Here's how the part is built. I have some questions about the finished solid (model axes, mm). Face numbers are marked on the shaded views. A direction names the side the tool comes from. Coordinates: 2 decimals unless noted, no trailing zeros. Write each loop counter-clockwise with the first axis right and the second up, starting at its lowest first coordinate (ties: lowest second). Pieces come first, ordered by that corner, then holes. Notation, with made-up numbers: (55.5, -36.5) -> (65.5, -36.5) arc R29 ccw to (65.5, 2.5) -> close; hole circle Ø6 at (30.5, 62.25). An arc over 180 degrees is marked (long way). Put each result on its own line as item: value. Start each with the question number.
Item 1: I want a section at C-C, the plane y = 33. List the corners of the cut face in (x, z) for me, then the cut area to 3 significant figures.
Item 2: If we mould it in two halves opening along X, with no side actions, what happens to the marked faces 1, 2 and 3? For each: released by +X, released by -X, zero draft, split by the parting line, or undercut.
Item 3: I want a section at D-D, the plane y = 109.5. State how many separate pieces and enclosed holes the cut face has, then the cut area to 3 significant figures.
Item 4: On a 3-axis mill with a long thin cutter (end or side, diameter ignored), from which of +Z, -Z, +X, -X, +Y, -Y can I reach the whole of each face in a straight line? I mean the marked faces 4, 5, 6, 7 and 8. Say none if no direction works.
Item 5: I want a section at B-B, the plane x = 0. List the corners of the cut face in (y, z) for me.
Item 6: I want a section at A-A, the plane z = 0. List the corners of the cut face in (x, y) for me.
Item 7: I need wall thicknesses on line 1 (Z direction, x = -29, y = 67.5); line 2 (X direction, y = 96, z = 9); line 3 (Y direction, x = 53.6, z = 0). Which ranges of each line are inside material? Lowest first, please. Write a range as [from, to].
Item 8: For pin 1 (21 mm diameter, centred on x = -39, z = 29.5, fed in from -Y); pin 2 (5 mm diameter, centred on x = 9, z = -22, fed in from -Y); pin 3 (4 mm diameter, centred on x = -42.5, z = -30.5, fed in from +Y); pin 4 (21.5 mm diameter, centred on y = 103.98, z = 0, fed in from +X), each with a flat end and sliding along its axis, tell me the tip position at first contact or that it passes through.
from build123d import *

# Parameters (mm, degrees)
SKETCH1_W           = 110
SKETCH1_H           = 90
SKETCH1_W_2         = 106
SKETCH1_H_2         = 86
BOSS_EXTRUDE1_DEPTH = 80
SKETCH2_W           = 110
SKETCH2_H           = 90
BOSS_EXTRUDE2_DEPTH = 2
BOSS_EXTRUDE3_DEPTH = 40
CUT_EXTRUDE1_DEPTH  = 40
BOSS_EXTRUDE4_DEPTH = 2
SKETCH11_W          = 23
SKETCH11_H          = 13
CUT_EXTRUDE2_DEPTH  = 13
REVOLVE_THIN3_ANGLE = 180
SKETCH13_R          = 12
CUT_EXTRUDE3_DEPTH  = 97
SKETCH14_R          = 12
CUT_EXTRUDE4_DEPTH  = 112


with BuildPart() as part:
    # Sketch1 → Boss-Extrude1 (new body)
    with BuildSketch(Plane(origin=(0, 0, 0), x_dir=(1, 0, 0), z_dir=(0, 1, 0))):
        Rectangle(SKETCH1_W, SKETCH1_H)
        Rectangle(SKETCH1_W_2, SKETCH1_H_2, mode=Mode.SUBTRACT)
    extrude(amount=BOSS_EXTRUDE1_DEPTH)

    # Sketch2 → Boss-Extrude2 (add)
    with BuildSketch(Plane(origin=(0, 80, 0), x_dir=(1, 0, 0), z_dir=(0, 1, 0))):
        Rectangle(SKETCH2_W, SKETCH2_H)
    extrude(amount=BOSS_EXTRUDE2_DEPTH)

    # Sketch3 → Boss-Extrude3 (add)
    with BuildSketch(Plane(origin=(0, 82, 0), x_dir=(1, 0, 0), z_dir=(0, 1, 0))):
        Polygon((55, 25.177973791), (24.883494565, 45), (-25.030734178, 45), (-55, 25.177973791), (-55, -24.883494565), (-24.436078892, -45), (24.883494565, -45), (55, -24.883494565), align=None)
        Polygon((53, 24.100004746), (24.284378107, 43), (-24.429161834, 43), (-53, 24.102910351), (-53, -23.805525521), (-23.836962434, -43), (24.27696917, -43), (53, -23.814274516), align=None, mode=Mode.SUBTRACT)
    extrude(amount=BOSS_EXTRUDE3_DEPTH)

    # Sketch7 → Cut-Extrude1 (cut)
    with BuildSketch(Plane(origin=(0, 82, 0), x_dir=(1, 0, 0), z_dir=(0, 1, 0))):
        Polygon((-24.429161834, 43), (-53, 24.102910351), (-53, -23.805525521), (-23.836962434, -43), (24.27696917, -43), (53, -23.814274516), (53, 24.100004746), (24.284378107, 43), align=None)
    extrude(amount=-CUT_EXTRUDE1_DEPTH, mode=Mode.SUBTRACT)

    # Sketch8 → Boss-Extrude4 (add)
    with BuildSketch(Plane(origin=(0, 122, 0), x_dir=(1, 0, 0), z_dir=(0, 1, 0))):
        Polygon((24.883494565, 45), (55, 25.177973791), (55, -24.883494565), (24.883494565, -45), (-24.436078892, -45), (-55, -24.883494565), (-55, 25.177973791), (-25.030734178, 45), align=None)
    extrude(amount=BOSS_EXTRUDE4_DEPTH)

    # Sketch11 → Cut-Extrude2 (cut)
    with BuildSketch(Plane(origin=(0, 124, 0), x_dir=(1, 0, 0), z_dir=(0, 1, 0))):
        Rectangle(SKETCH11_W, SKETCH11_H)
    extrude(amount=-CUT_EXTRUDE2_DEPTH, mode=Mode.SUBTRACT)

    # Sketch12 → Revolve-Thin3 (revolve)
    with BuildSketch(Plane(origin=(0, 124, 0), x_dir=(1, 0, 0), z_dir=(0, 1, 0))):
        with BuildLine():
            ThreePointArc((-43.995827048, 0), (0, -43.995827048), (43.995827048, 0))
            Line((43.995827048, 0), (41.995827048, 0))
            ThreePointArc((41.995827048, 0), (0, -41.995827048), (-41.995827048, 0))
            Line((-41.995827048, 0), (-43.995827048, 0))
        make_face()
    revolve(axis=Axis((43.995827048, 124, 0), (-1, 0, 0)), revolution_arc=REVOLVE_THIN3_ANGLE)

    # Sketch13 → Cut-Extrude3 (cut)
    with BuildSketch(Plane(origin=(0, 0, -45), x_dir=(-1, 0, 0), z_dir=(0, 0, -1))):
        with Locations((0, 101.721715456)):
            Circle(SKETCH13_R)
    extrude(amount=-CUT_EXTRUDE3_DEPTH, mode=Mode.SUBTRACT)

    # Sketch14 → Cut-Extrude4 (cut)
    with BuildSketch(Plane.ZY.offset(55)):
        with Locations((0, 103.980631389)):
            Circle(SKETCH14_R)
    extrude(amount=-CUT_EXTRUDE4_DEPTH, mode=Mode.SUBTRACT)


solid = part.part
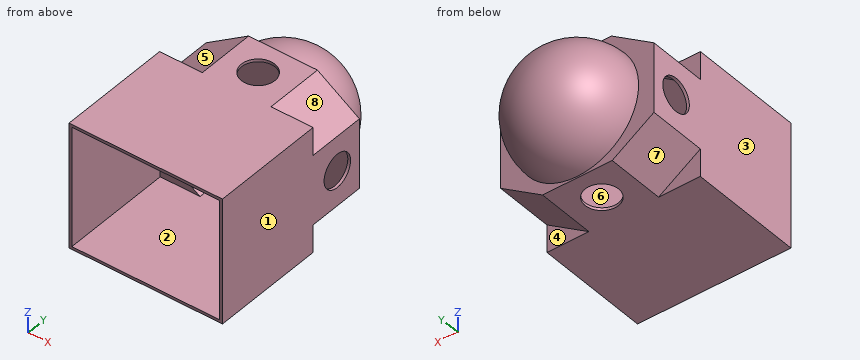
Calculated:
1. outline: (-55, -45) -> (55, -45) -> (55, 45) -> (-55, 45) -> close; hole (-53, -43) -> (53, -43) -> (53, 43) -> (-53, 43) -> close
1. area: 784 mm2
2. face 1: released by +X
2. face 2: undercut
2. face 3: released by -X
3. separate pieces: 4
3. enclosed holes: 0
3. area: 517 mm2
4. face 4: -Z, +X, +Y
4. face 5: +Z, -X, +Y
4. face 6: -Y
4. face 7: -Z, -X, +Y
4. face 8: +Z, +X, +Y
5. outline: (0, -45) -> (89.72, -45) -> (89.72, -43) -> (0, -43) -> close; (0, 43) -> (89.72, 43) -> (89.72, 45) -> (0, 45) -> close; (113.72, -45) -> (124, -45) -> (124, -44) arc R44 ccw to (124, 44) -> (124, 45) -> (113.72, 45) -> (113.72, 43) -> (122, 43) -> (122, 6.5) -> (124, 6.5) -> (124, 42) arc R42 cw to (124, -42) -> (124, -6.5) -> (122, -6.5) -> (122, -43) -> (113.72, -43) -> close
6. outline: (-55, 0) -> (-53, 0) -> (-53, 91.98) -> (-55, 91.98) -> close; (-55, 115.98) -> (-53, 115.98) -> (-53, 122) -> (-11.5, 122) -> (-11.5, 124) -> (-42, 124) arc R42 cw to (42, 124) -> (11.5, 124) -> (11.5, 122) -> (53, 122) -> (53, 115.98) -> (55, 115.98) -> (55, 124) -> (44, 124) arc R44 ccw to (-44, 124) -> (-55, 124) -> close; (53, 0) -> (55, 0) -> (55, 91.98) -> (53, 91.98) -> close
7. line 1: z = [-45, -43], [43, 45]
7. line 2: x = [-55, -53], [53, 55]
7. line 3: y = [0, 91.98], [115.98, 124]
8. pin 1: stops at y = 80
8. pin 2: stops at y = 122
8. pin 3: stops at y = 124
8. pin 4: passes through
